The figure shows three views and two pictorial views of one solid part (mm, origin at its lowest corner). Answer the questions. A direction names the side the tool comes from. Coordinates: 2 decimals unless noted, no trailing zeros. Loops run counter-clockwise (first coordinate to the right, second up) from the corner with the lowest first, then second, coordinate; pieces in that order, holes last. Notation, with made-up numbers: M 83.5,-32 L 123.5,-32 A22 cw 123.5,-21 Z; hole C 87.25,35 d2. An arc over 180 degrees is marked long. Write each question's results on one line, items separated by ' | '.
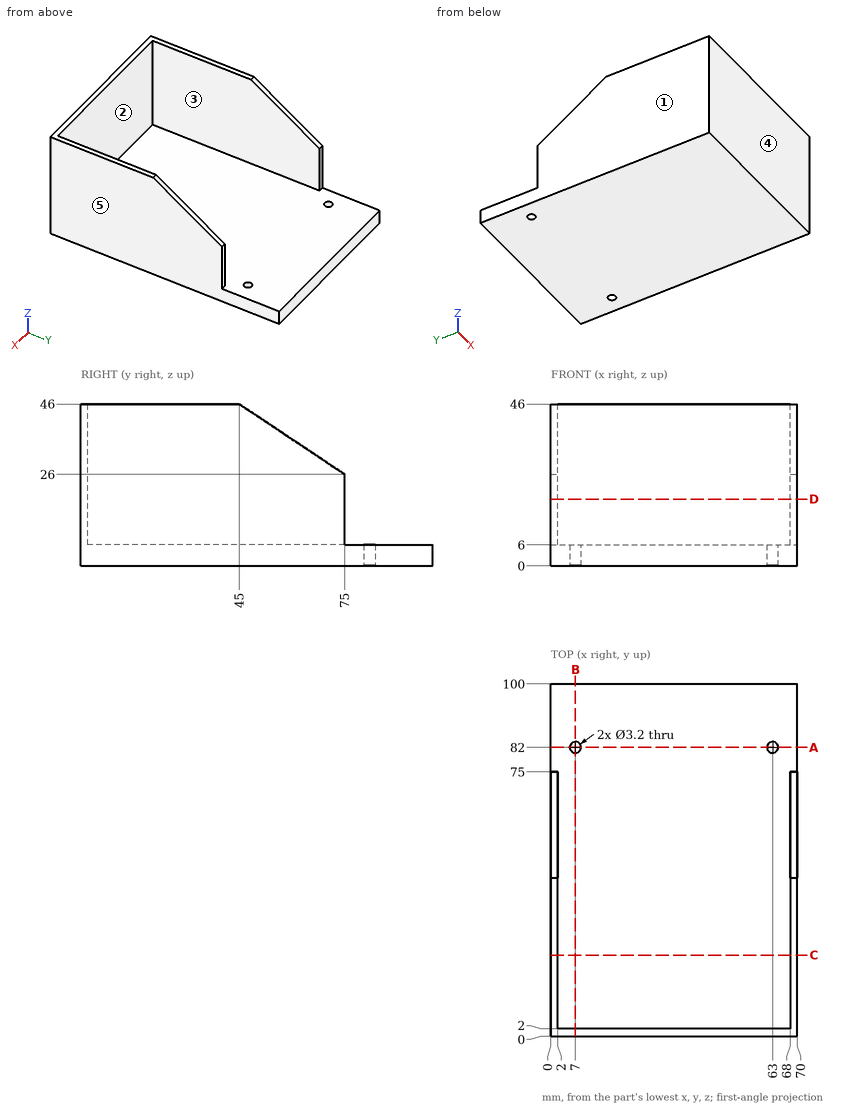
1) Find section C-C, the plane y = 23. Give the vertices of the cut face in (x, z), and give its area (3 significant figures).
Check result:
outline: M 0,0 L 70,0 L 70,46 L 68,46 L 68,6 L 2,6 L 2,46 L 0,46 Z | area: 580 mm^2
2) Given pin 1 Ø0.6 at (x, z) = (68.5, 20) entering from +Y; pin 2 Ø12 at (x, y) = (51, 24.5) entering from +Z; pin 3 Ø4 at (x, z) = (13.5, 14) entering from +Y, each flat-ended and moving along its own axis, determine where each tip first touches the part or whether it passes through.
Check result:
pin 1: y = 75 | pin 2: z = 6 | pin 3: y = 2
3) Straight lines are drawn through the part: probe 1 along X at (y, z) = (82, 4.35); probe 2 along X at (y, z) = (62, 34); probe 3 along Y at (x, z) = (63, 3). For each, find the intervals that lie inside material, in ascending order. Write a range as [from, to].
Check result:
probe 1: [0, 5.4], [8.6, 61.4], [64.6, 70] | probe 2: [0, 2], [68, 70] | probe 3: [0, 80.4], [83.6, 100]
4) For a pull along X with two mould halves and no side action, classify the marked faces 3, 4 and 5 as released by +X, released by -X, zero draft, split by the parting line, or undercut.
Check result:
face 3: undercut | face 4: zero draft | face 5: released by +X
5) Find section D-D, the plane z = 19. Give the vertices of the cut face in (x, y), and give its area (3 significant figures).
Check result:
outline: M 0,0 L 70,0 L 70,75 L 68,75 L 68,2 L 2,2 L 2,75 L 0,75 Z | area: 432 mm^2
6) Find section B-B, the plane x = 7. Give the vertices of the cut face in (y, z).
Check result:
outline: M 0,0 L 80.4,0 L 80.4,6 L 2,6 L 2,46 L 0,46 Z; M 83.6,0 L 100,0 L 100,6 L 83.6,6 Z
7) Find section A-A, the plane y = 82. Give the vertices of the cut face in (x, z).
Check result:
outline: M 0,0 L 5.4,0 L 5.4,6 L 0,6 Z; M 8.6,0 L 61.4,0 L 61.4,6 L 8.6,6 Z; M 64.6,0 L 70,0 L 70,6 L 64.6,6 Z
8) Which of the six approach directions +Z, -Z, +X, -X, +Y, -Y give full straight-line access (tool end or side, diameter ignored) to the marked faces 1 and 2?
Check result:
face 1: +Z, -Z, -X, +Y, -Y | face 2: +Z, +Y
